Geometry: final body of the model. Coordinates: model frame, mm. A direction names the side the tool comes from. Give positions to 0.01 mm unless a question says otherwise; leave off trailing zeros. Write each loop counter-clockwise with the first axis right and the second up, starting at its lowest first coordinate (ties: lowest second). Pieces come first, ordered by that corner, then holes.
from build123d import *
from OCP.BRepFilletAPI import BRepFilletAPI_MakeChamfer

# Parameters (mm, degrees)
BOSS_EXTRUDE1_DEPTH = 9.5
SKETCH2_R           = 2
CUT_EXTRUDE1_DEPTH  = 44
CHAMFER3_SIZE       = 2.31
CHAMFER3_SIZE2      = 2.75
CHAMFER4_SIZE       = 2.75
CHAMFER4_SIZE2      = 2.31
FILLET2_R           = 2
FILLET3_R           = 10
FILLET4_R           = 8
CHAMFER5_SIZE       = 0.3


with BuildPart() as part:
    # Sketch1 → Boss-Extrude1 (new body)
    with BuildSketch(Plane.XY):
        Polygon((25.25, -9.5), (37.25, -9.5), (37.25, 7), (25.25, 7), (-11.25, 17.5), (-37.25, 17.5), (-37.25, 10.5), (-19.25, 10.5), (-19.25, -10.5), (-37.25, -10.5), (-37.25, -17.5), (-11.25, -17.5), (-4.75, -3.5), (20.25, -3.5), align=None)
    extrude(amount=BOSS_EXTRUDE1_DEPTH)

    # Sketch2 → Cut-Extrude1 (cut)
    with BuildSketch(Plane.XZ.offset(17.5)):
        with Locations(Location((-32.5, 4.75, 0), (0, 0, 270))):
            Circle(SKETCH2_R)
        with Locations((32.5, 4.75)):
            Circle(SKETCH2_R)
    extrude(amount=-CUT_EXTRUDE1_DEPTH, mode=Mode.SUBTRACT)

    # Chamfer3: one chamfer whose edges measure the first distance from different faces: ONE call of the kernel's chamfer builder (chamfer() names one face for all edges)
    chamfer3_edges_1 = [part.edges().sort_by_distance(p)[0] for p in [
        (-37.25, -14, 0),
        (-37.25, 14, 0),
    ]]
    chamfer3_side_1 = [part.faces().sort_by_distance(p)[0] for p in [
        (-1.759689035, 1.451005524, 0),
    ]]
    chamfer3_edges_2 = [part.edges().sort_by_distance(p)[0] for p in [
        (37.25, -1.25, 9.5),
    ]]
    chamfer3_side_2 = [part.faces().sort_by_distance(p)[0] for p in [
        (-1.759689035, 1.451005524, 9.5),
    ]]
    chamfer3 = BRepFilletAPI_MakeChamfer(part.part.solid().wrapped)
    for e in chamfer3_edges_1:
        chamfer3.Add(CHAMFER3_SIZE, CHAMFER3_SIZE2, e.wrapped, chamfer3_side_1[0].wrapped)  # the first distance lies on this face
    for e in chamfer3_edges_2:
        chamfer3.Add(CHAMFER3_SIZE, CHAMFER3_SIZE2, e.wrapped, chamfer3_side_2[0].wrapped)  # the first distance lies on this face
    add(Compound.cast(chamfer3.Shape()), mode=Mode.REPLACE)

    # Chamfer4: one chamfer whose edges measure the first distance from different faces: ONE call of the kernel's chamfer builder (chamfer() names one face for all edges)
    chamfer4_edges_1 = [part.edges().sort_by_distance(p)[0] for p in [
        (-37.25, 14, 9.5),
    ]]
    chamfer4_side_1 = [part.faces().sort_by_distance(p)[0] for p in [
        (-37.25, 14, 6.125),
    ]]
    chamfer4_edges_2 = [part.edges().sort_by_distance(p)[0] for p in [
        (37.25, -1.25, 0),
    ]]
    chamfer4_side_2 = [part.faces().sort_by_distance(p)[0] for p in [
        (37.25, -1.25, 3.375),
    ]]
    chamfer4_edges_3 = [part.edges().sort_by_distance(p)[0] for p in [
        (-37.25, -14, 9.5),
    ]]
    chamfer4_side_3 = [part.faces().sort_by_distance(p)[0] for p in [
        (-37.25, -14, 6.125),
    ]]
    chamfer4 = BRepFilletAPI_MakeChamfer(part.part.solid().wrapped)
    for e in chamfer4_edges_1:
        chamfer4.Add(CHAMFER4_SIZE, CHAMFER4_SIZE2, e.wrapped, chamfer4_side_1[0].wrapped)  # the first distance lies on this face
    for e in chamfer4_edges_2:
        chamfer4.Add(CHAMFER4_SIZE, CHAMFER4_SIZE2, e.wrapped, chamfer4_side_2[0].wrapped)  # the first distance lies on this face
    for e in chamfer4_edges_3:
        chamfer4.Add(CHAMFER4_SIZE, CHAMFER4_SIZE2, e.wrapped, chamfer4_side_3[0].wrapped)  # the first distance lies on this face
    add(Compound.cast(chamfer4.Shape()), mode=Mode.REPLACE)

    # Fillet2
    fillet2_edges = [part.edges().sort_by_distance(p)[0] for p in [
        (-19.25, -10.5, 4.75),
        (-19.25, 10.5, 4.75),
    ]]
    fillet(fillet2_edges, radius=FILLET2_R)

    # Fillet3
    fillet3_edges = [part.edges().sort_by_distance(p)[0] for p in [
        (25.25, 7, 4.75),
        (20.25, -3.5, 4.75),
        (-4.75, -3.5, 4.75),
        (-11.25, -17.5, 4.75),
        (-11.25, 17.5, 4.75),
    ]]
    fillet(fillet3_edges, radius=FILLET3_R)

    # Fillet4
    fillet4_edges = [part.edges().sort_by_distance(p)[0] for p in [
        (25.25, -9.5, 4.75),
    ]]
    fillet(fillet4_edges, radius=FILLET4_R)

    # Chamfer5
    chamfer5_edges = [part.edges().sort_by_distance(p)[0] for p in [
        (-19.835786438, -9.914213562, 0),
        (-19.835786438, -9.914213562, 9.5),
        (-19.835786438, 9.914213562, 0),
        (-19.835786438, 9.914213562, 9.5),
        (-8, -10.5, 0),
        (-8, -10.5, 9.5),
        (8.599321356, -3.5, 0),
        (7, 12.25, 0),
        (-11.263803813, 17.402084612, 0),
        (-12.252388949, -15.929446324, 0),
        (8.599321356, -3.5, 9.5),
        (7, 12.25, 9.5),
        (-11.263803813, 17.402084612, 9.5),
        (-12.252388949, -15.929446324, 9.5),
        (-3.747611051, -5.070553676, 0),
        (-3.747611051, -5.070553676, 9.5),
        (19.648733445, -4.371290708, 9.5),
        (25.263803813, 7.097915388, 0),
        (25.263803813, 7.097915388, 9.5),
        (19.648733445, -4.371290708, 0),
        (25.716672081, -8.802967433, 0),
        (25.716672081, -8.802967433, 9.5),
        (30.5, -9.5, 4.75),
        (30.5, 7, 4.75),
        (-28.095, 10.5, 0),
        (-26.286196086, -17.5, 0),
        (-28.095, -10.5, 0),
        (-23.799884776, 17.5, 0),
        (31.961329203, -9.5, 9.5),
        (30.799884776, 7, 9.5),
        (30.799884776, 7, 0),
        (31.961329203, -9.5, 0),
        (-23.799884776, 17.5, 9.5),
        (-28.095, 10.5, 9.5),
        (-28.095, -10.5, 9.5),
        (-26.286196086, -17.5, 9.5),
        (-19.25, 0, 0),
        (-19.25, 0, 9.5),
    ]]
    chamfer(chamfer5_edges, length=CHAMFER5_SIZE)


solid = part.part
Q1. Section A-A on x = -29. Output: boundary loops of the cut face in (y, z).
Filled sheet:
outline: (-17.5, 0.3) - (-17.2, 0) - (-10.8, 0) - (-10.5, 0.3) - (-10.5, 9.2) - (-10.8, 9.5) - (-17.2, 9.5) - (-17.5, 9.2) - close; (10.5, 0.3) - (10.8, 0) - (17.2, 0) - (17.5, 0.3) - (17.5, 9.2) - (17.2, 9.5) - (10.8, 9.5) - (10.5, 9.2) - close
Q2. Section C-C on z = 4.75. Count the separate pieces of the cut face and the enclosed holes in it, plus the area to 3 significant figures.
Filled sheet:
separate pieces: 4
enclosed holes: 0
area: 1,250 mm2
Q3. Access query for faces 1 (the conical face through (-3.88, -5.01, 9.32)), 2 (the conical face through (-3.877, -5.018, 0.185)), 3 (the cylindrical face through (-19.82, -9.9, 4.81)), 4 (the cylindrical face through (-3.81, -5.11, 4.81)), 5 (the conical face through (-19.768, 10.015, 9.319)). Directions: +Z, -Z, +X, -X, +Y, -Y. A direction counts if a zero-diameter tool reaches every point of the face in a straight line with its end or side. Return the directions, or none.
Filled sheet:
face 1: +Z, -Y
face 2: -Z, -Y
face 3: +Z, -Z, -X
face 4: +Z, -Z, -Y
face 5: +Z, -X
Q4. Pin query (flat end, axial travel): P1, Ø2, axis at x = -8, y = -13.5, coming from the -Z side; P2, Ø4.5, axis at y = -0.5, z = 6.5, coming from the -X side; P3, Ø3, axis at y = 8.5, z = 6.5, coming from the -X side; P4, Ø5, axis at x = 32.5, z = 4.75, coming from the -Y side. Return the tip coordinate at first contact, or that it passes through.
Filled sheet:
P1: passes through
P2: stops at x = -19.25
P3: stops at x = -19.93
P4: stops at y = -9.5
Q5. Section B-B on y = 4. Output: boundary loops of the cut face in (x, z), plus the area to 3 significant figures.
Filled sheet:
outline: (-19.25, 0.3) - (-18.95, 0) - (34.94, 0) - (37.25, 2.75) - (37.25, 6.75) - (34.94, 9.5) - (-18.95, 9.5) - (-19.25, 9.2) - close; hole circle Ø4 at (32.5, 4.75)
area: 518 mm2
Q6. Section D-D on x = 32.5. Output: boundary loops of the cut face in (y, z), plus the area to 3 significant figures.
Filled sheet:
outline: (-9.5, 0.3) - (-9.2, 0) - (6.7, 0) - (7, 0.3) - (7, 2.45) - (6.7, 2.75) - (-9.2, 2.75) - (-9.5, 2.45) - close; (-9.5, 7.05) - (-9.2, 6.75) - (6.7, 6.75) - (7, 7.05) - (7, 9.2) - (6.7, 9.5) - (-9.2, 9.5) - (-9.5, 9.2) - close
area: 90.4 mm2
Q7. Pull-direction query (X, two-part tool) for faces 6 (the flat face through (-37.25, -14, 5)), 7 (the flat face through (0, 0, 9.5)), 8 (the cylindrical face through (34.408, -1.361, 5.351)); classes: released by +X, released by -X, zero draft, split by the parting line, or undercut.
Filled sheet:
face 6: released by -X
face 7: zero draft
face 8: undercut
Q8. Ray query, line 1 along Y through (x, z) = (-27, 1.5); line 2 along X through (y, z) = (-14.75, 4.75); line 3 along X through (y, z) = (-12, 4.75). Return the intervals inside material, ascending.
Filled sheet:
line 1: y = -17.5 to -10.5, 10.5 to 17.5
line 2: x = -37.25 to -34.5, -30.5 to -10.74
line 3: x = -37.25 to -34.5, -30.5 to -8.7
